```python
from build123d import *

# Parameters (mm, degrees)
SKETCH2_W           = 127.41
SKETCH2_H           = 75.848
SKETCH2_R           = 5.8
SKETCH2_R_2         = 1.975434392
SKETCH2_R_3         = 2.02059866
SKETCH2_R_4         = 2.005784304
SKETCH2_R_5         = 2.007647525
SKETCH2_W_2         = 2
SKETCH2_H_2         = 23.848
SKETCH2_W_3         = 45.41
SKETCH2_H_3         = 2
BOSS_EXTRUDE1_DEPTH = 2


with BuildPart() as part:
    # Sketch2 → Boss-Extrude1 (new body)
    with BuildSketch(Plane(origin=(0, 0, 0), x_dir=(1, 0, 0), z_dir=(0, 1, 0))):
        with Locations((56.48154317, 30.702122774)):
            Rectangle(SKETCH2_W, SKETCH2_H)
        with Locations(Location((92.113682499, 29.850625922, 0), (0, 0, 270))):
            Circle(SKETCH2_R, mode=Mode.SUBTRACT)
        with Locations(Location((92.113682499, 11.563322273, 0), (0, 0, 270))):
            Circle(SKETCH2_R, mode=Mode.SUBTRACT)
        with Locations(Location((92.131948628, 46.863483745, 0), (0, 0, 270))):
            Circle(SKETCH2_R, mode=Mode.SUBTRACT)
        with Locations(Location((3.695346689, 3.585176853, 0), (0, 0, 270))):
            Circle(SKETCH2_R_2, mode=Mode.SUBTRACT)
        with Locations(Location((3.945209928, 57.606557407, 0), (0, 0, 270))):
            Circle(SKETCH2_R_3, mode=Mode.SUBTRACT)
        with Locations(Location((109.903070514, 57.08563935, 0), (0, 0, 270))):
            Circle(SKETCH2_R_4, mode=Mode.SUBTRACT)
        with Locations(Location((109.140500171, 3.238215507, 0), (0, 0, 270))):
            Circle(SKETCH2_R_5, mode=Mode.SUBTRACT)
        with Locations((-2.22345683, 30.702122774)):
            Rectangle(SKETCH2_W_2, SKETCH2_H_2, mode=Mode.SUBTRACT)
        with Locations((56.48154317, 63.626122774)):
            Rectangle(SKETCH2_W_3, SKETCH2_H_3, mode=Mode.SUBTRACT)
        with Locations((115.18654317, 30.702122774)):
            Rectangle(SKETCH2_W_2, SKETCH2_H_2, mode=Mode.SUBTRACT)
        with Locations((56.48154317, -2.221877226)):
            Rectangle(SKETCH2_W_3, SKETCH2_H_3, mode=Mode.SUBTRACT)
    extrude(amount=BOSS_EXTRUDE1_DEPTH)


solid = part.part
```
For this review, take the finished solid that the model builds, in its own axes (mm). Coordinates: 2 decimals unless noted, no trailing zeros. Write each loop counter-clockwise with the first axis right and the second up, starting at its lowest first coordinate (ties: lowest second). Pieces come first, ordered by that corner, then holes. Notation, with made-up numbers: (80.5, 6.5) -> (92.5, 6.5) arc R26 cw to (92.5, 35.5) -> close; hole circle Ø11 at (29, 78.5). An arc over 180 degrees is marked (long way). Put each result on its own line as item: value.
Q1. The part is to be moulded in two halves that separate along X. For faces 1 (the cylindrical face through (5.654, 0.986, -3.842)), 2 (the flat face through (56, 0, -31)), say which applies: +X half, -X half, draft (parallel to the pull), parting line (faces both ways), or undercut.
From the geometry:
face 1: undercut
face 2: draft
Q2. Take a section at C-C, the plane y = 1.3. Count the separate pieces of the cut face and the enclosed holes in it, then the cut area to 3 significant figures.
From the geometry:
separate pieces: 1
enclosed holes: 11
area: 9,020 mm2
Q3. Take a section at D-D, the plane z = -50.5. State the section outline as (x, y) points.
From the geometry:
outline: (-7.22, 0) -> (87.61, 0) -> (87.61, 2) -> (-7.22, 2) -> close; (96.65, 0) -> (120.19, 0) -> (120.19, 2) -> (96.65, 2) -> close
Q4. Wall thickness on L1, parallel to X at y = 1.45, z = -39; L2, parallel to Z at x = 74, y = 1.8; L3, parallel to X at y = 1.65, z = -47: over which ranges is each line inside the solid? List them lowest first.
From the geometry:
L1: x = -7.22 to -3.22, -1.22 to 114.19, 116.19 to 120.19
L2: z = -68.63 to -64.63, -62.63 to 1.22, 3.22 to 7.22
L3: x = -7.22 to 86.33, 97.93 to 120.19
Q5. Take a section at A-A, the plane z = -22.5. State the section outline as (x, y) points, then the cut area to 3 significant figures.
From the geometry:
outline: (-7.22, 0) -> (-3.22, 0) -> (-3.22, 2) -> (-7.22, 2) -> close; (-1.22, 0) -> (114.19, 0) -> (114.19, 2) -> (-1.22, 2) -> close; (116.19, 0) -> (120.19, 0) -> (120.19, 2) -> (116.19, 2) -> close
area: 247 mm2
Q6. Take a section at B-B, the plane x = 41. State the section outline as (y, z) points, then the cut area to 3 significant figures.
From the geometry:
outline: (0, -68.63) -> (2, -68.63) -> (2, -64.63) -> (0, -64.63) -> close; (0, -62.63) -> (2, -62.63) -> (2, 1.22) -> (0, 1.22) -> close; (0, 3.22) -> (2, 3.22) -> (2, 7.22) -> (0, 7.22) -> close
area: 144 mm2
